Autodesk Inventor part; units mm, degrees
ref_plane "Work Plane1" through (1.525, 0, 0) normal (0, 0, 1) x (1, 0, 0)
ref_plane "YZ Plane" through (0, 0, 0) normal (1, 0, 0) x (0, 1, 0)
ref_plane "XZ Plane" through (0, 0, 0) normal (0, 1, 0) x (-1, 0, 0)
sketch "Sketch1" plane through (0, 0, 0) normal (0, 0, 1) x (1, 0, 0)
  line L0 (0, 12.67) -> (0, 9)
  line L1 (7.5, 9) -> (35, 9)
  line L2 (35, 9) -> (35, 0)
  line L3 (35, 0) -> (-0.8001, 0)
  line L4 (-7.9601, 0) -> (42.16, 0)
  line L5 (-0.8001, 0) -> (-0.8001, 12.67)
  line L6 (-0.8001, 12.67) -> (0, 12.67)
  line L7 (7.5, 9) -> (5.9663, 9)
  line L8 (5.9663, 9) -> (0, 9)
  line L9 (0, -2.534) -> (0, 15.204)
  dimension "d0" = 35
  dimension "d1" = 27.5
  dimension "d2" = 18
  dimension "d9" = 0.8001
  dimension "d10" = 25.34
  dimension "d13" = 1.5337
  dimension "d14" = 18
revolve "Body" add sketch "Sketch1" angle 360 about axis through (35, 0, 0) along (-1, 0, 0)
sketch "Sketch2" plane through (-0.8001, 0, 0) normal (-1, 0, 0) x (0, 0, 1)
  line L0 (0, 15.5885) -> (13.5, 7.7942)
  line L1 (13.5, 7.7942) -> (13.5, -7.7942)
  line L2 (13.5, -7.7942) -> (0, -15.5885)
  line L3 (0, -15.5885) -> (-13.5, -7.7942)
  line L4 (-13.5, -7.7942) -> (-13.5, 7.7942)
  line L5 (-13.5, 7.7942) -> (0, 15.5885)
  point P0 (0, 0)
  point P1 (0, 0)
  dimension "d11" = 27
extrude "Head" add sketch "Sketch2" along normal blind 10.7
sketch "Sketch4" plane through (0, 0, 0) normal (0, 0, 1) x (1, 0, 0)
  line L0 (-11.5001, 13.5) -> (-11.5001, 15.5885)
  line L1 (-11.5001, 15.5885) -> (-10.2943, 15.5885)
  line L2 (-10.2943, 15.5885) -> (-11.5001, 13.5)
  line L3 (-13.6401, 0) -> (1.3399, 0)
  line L4 (-0.8001, 15.5885) -> (-11.5001, 15.5885)
  line L5 (-11.5001, 7.7942) -> (-11.5001, 15.5885)
  dimension "d5" = 30
  dimension "d19" = 27
revolve "Chamfer1" cut sketch "Sketch4" angle 360 about axis through (-10, 0, 0) along (1, 0, 0)
thread "Thread"
chamfer "Chamfer2" distance 1.5336 distance2 1.5337 1 edges at (35, -9, 0) measured on face at (35, 1.0638, -2.805)
ref_plane "Work Plane1" through (1.525, 0, 0) normal (0, 0, 1) x (1, 0, 0)
equation "\"d0\" = NLG"
equation "\"d1\" = GEL"
equation "\"d2\" = GD"
equation "\"d10\" = SD2"
equation "\"d14\" = BDM"
equation "\"d11\" = SW"
equation "\"d3\" = KOH - SD"
equation "\"d5\" = ANG1"
equation "\"d19\" = SW0"
equation "\"d15\" = GEL"
equation "\"d6\" = -0.5 * SPD + 0.5 * GD"
equation "\"NLG\" = 35"
equation "\"GD\" = NND"
equation "\"BDM\" = NND"
equation "\"KOH\" = 11.5"
equation "\"GEL\" = 27.5"
equation "\"SW\" = 27"
equation "\"SW0\" = SW"
equation "\"SPD\" = NND - 1.2269 * PTC"
equation "\"SD2\" = 25.34"
equation "\"SD\" = 0.8"
equation "\"ANG1\" = 30deg"
equation "\"GAL\" = 0.61345 * PTC"
equation "\"GUL\" = 0.61345 * PTC"
equation "\"RR\" = 0.6"
equation "\"GD1\" = THREADDIA - 1.2269 * PTC"
equation "\"THREADDIA\" = 18"
equation "\"SDH\" = SD2"
equation "\"SDHG\" = 7.5"
equation "\"TOA\" = 30deg"
equation "\"PTC\" = 2.5"
equation "\"NND\" = 18"
equation "\"E0\" = 31.185"
properties part number "ISO 4017 - M18 x 35" material "Stainless Steel, 440C"
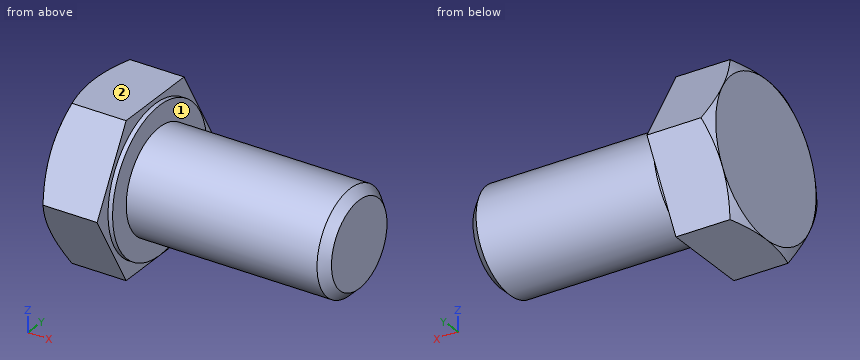
Source: CAD feature listing. Evaluate the final solid. Frame: model axes, mm. Face numbers are marked on the shaded views. A direction names the side the tool comes from. Give positions to 0.01 mm unless a question says otherwise; leave off trailing zeros. Order: outer loops, then holes, each group sorted by start corner. A loop starts at its lowest first (then second) coordinate and runs counter-clockwise, first axis right, second up. Notation, with made-up numbers: (-15, 22.25) -> (36, 22.25) arc R18 cw to (36, 36.25) -> close; hole circle Ø4 at (65, -37). An arc over 180 degrees is marked (long way). Use a Markdown table: item, result.
1) Contact query for flat-ended pins moving along their axis: P1, Ø4, axis at x = 3, y = -5.5, coming from the +Z side; P2, Ø5, axis at y = -7.5, z = -8, coming from the +X side; P3, Ø1, axis at x = 19.5, z = 5.5, coming from the +Y side. Output: stop coordinate, or through.
Answer list:
| item | result |
|---|---|
| P1 | z = 8.29 |
| P2 | x = 34 |
| P3 | y = 7.48 |
2) Reachability of the marked faces 1 and 2 from +Z, -Z, +X, -X, +Y, -Y: full face, straight path, thin tool, end or side. Return the list, or none.
Answer list:
| item | result |
|---|---|
| face 1 | +X |
| face 2 | +Z, +X, -X, +Y, -Y |
3) Section query A-A, the plane x = 31. Return the cut outline in (y, z), then the cut area to 3 significant figures.
Answer list:
| item | result |
|---|---|
| outline | circle Ø18 at (0, 0) |
| area | 254 mm² |
4) Ray query, line 1 along X through (y, z) = (8, 9.5); line 2 along X through (y, z) = (-9, -9.75); line 3 along Z through (x, y) = (29, 5). Return the intervals inside material, ascending. Write a range as [from, to].
Answer list:
| item | result |
|---|---|
| line 1 | [-11.5, 0] |
| line 2 | [-11.5, -0.8] |
| line 3 | [-7.48, 7.48] |
